Solid Edge part; units mm, degrees
sketch "Sketch1" plane through (0, 0, 0) normal (0, 0, 1) x (1, 0, 0)
  line L0 (45, 22.5) -> (-45, 22.5)
  line L1 (-45, -22.5) -> (45, -22.5)
  arc A0 (-45, -22.5) -> (-45, 22.5) centre (-45, 0) cw
  arc A1 (45, 22.5) -> (45, -22.5) centre (45, 0) cw
  circle A2 centre (-45, 0) radius 10
  circle A3 centre (45, 0) radius 10
extrude "Protrusion1" add sketch "Sketch1" against normal blind 15
sketch "Sketch2" plane through (0, 0, 0) normal (1, 0, 0) x (0, 1, 0)
  line L0 (-7.5, 55) -> (-22.5, 0)
  line L1 (-22.5, 0) -> (0, 0)
  line L2 (0, 0) -> (0, 55)
  line L3 (0, 55) -> (-7.5, 55)
extrude "ExtrudedProtrusion_2" add sketch "Sketch2" along normal mid plane 15
sketch "Sketch3" plane through (0, 0, 0) normal (0, -1, 0) x (1, 0, 0)
  line L0 (15, 55) -> (24.5, 0)
  line L1 (0, 0) -> (24.5, 0)
  line L2 (0, 0) -> (-24.5, 0)
  line L3 (-15, 55) -> (-24.5, 0)
  line L4 (0, 55) -> (-15, 55)
  line L5 (0, 55) -> (15, 55)
extrude "ExtrudedProtrusion_3" add sketch "Sketch3" against normal blind 22.5
sketch "Sketch4" plane through (0, 7.5, 55) normal (0, 0, 1) x (0, 1, 0)
  line L0 (-15, 15) -> (-15, -15)
  line L1 (-15, -15) -> (15, -15)
  line L2 (15, -15) -> (15, 15)
  line L3 (15, 15) -> (-15, 15)
extrude "ExtrudedProtrusion_4" add sketch "Sketch4" along normal blind 30
sketch "Sketch5" plane through (0, -7.5, 70) normal (0, -1, 0) x (1, 0, 0)
  line L0 (10, -10) -> (10, 10)
  line L1 (10, 10) -> (-10, 10)
  line L2 (-10, 10) -> (-10, -10)
  line L3 (-10, -10) -> (10, -10)
extrude "ExtrudedCutout_1" cut sketch "Sketch5" along normal mid plane 100
sketch "Sketch6" plane through (15, 7.5, 70) normal (1, 0, 0) x (0, 1, 0)
  line L0 (5, -12) -> (5, 12)
  line L1 (5, 12) -> (-5, 12)
  line L2 (-5, 12) -> (-5, -12)
  line L3 (-5, -12) -> (5, -12)
extrude "ExtrudedProtrusion_5" add sketch "Sketch6" along normal blind 25
sketch "Sketch7" plane through (-15, 7.5, 70) normal (-1, 0, 0) x (0, 0, 1)
  line L0 (-12, 5) -> (12, 5)
  line L1 (12, 5) -> (12, -5)
  line L2 (12, -5) -> (-12, -5)
  line L3 (-12, -5) -> (-12, 5)
extrude "ExtrudedProtrusion_6" add sketch "Sketch7" along normal blind 25
sketch "Sketch8" plane through (27.5, 2.5, 70) normal (0, -1, 0) x (1, 0, 0)
  circle A0 centre (12.5, 0) radius 5
extrude "ExtrudedCutout_3" cut sketch "Sketch8" along normal mid plane 50
sketch "Sketch9" plane through (27.5, 2.5, 70) normal (0, -1, 0) x (1, 0, 0)
  circle A0 centre (12.5, 0) radius 12
  circle A1 centre (12.5, 0) radius 5
extrude "ExtrudedProtrusion_7" add sketch "Sketch9" against normal blind 10
sketch "Sketch10" plane through (-27.5, 2.5, 70) normal (0, -1, 0) x (1, 0, 0)
  circle A0 centre (-12.5, 0) radius 12
  circle A1 centre (-12.5, 0) radius 5
extrude "ExtrudedProtrusion_8" add sketch "Sketch10" against normal blind 10
sketch "Sketch11" plane through (-27.5, 2.5, 70) normal (0, -1, 0) x (1, 0, 0)
  circle A0 centre (-12.5, 0) radius 5
extrude "ExtrudedCutout_5" cut sketch "Sketch11" along normal mid plane 50
fillet "Round_2" radius 3 4 edges at (15, 7.5, 82) (-15, 7.5, 82) (15, 7.5, 58) (-15, 7.5, 58)
Here's how the part is built. I have some questions about the finished solid (model axes, mm). A direction names the side the tool comes from. Coordinates: 2 decimals unless noted, no trailing zeros. Loops run counter-clockwise (first coordinate to the right, second up) from the corner with the lowest first, then second, coordinate; pieces in that order, holes last. Notation, with made-up numbers: (30, -2.75) -> (41, -2.75) arc R23 cw to (41, 29.25) -> close; hole circle Ø11 at (-5.5, -5). An arc over 180 degrees is marked (long way). Use one line per item in the form item = value. Start each with the question number.
(1) We'd pull the mould along X, two halves only. Please class faces 4 (the face through (-15, 1, 70)), 5 (the face through (-10, 8, 70)), 6 (the face through (33, 2.5, 70)): pulls with the +X half, pulls with the -X half, needs draft (parallel to the pull), parting line crosses it, or undercut.
(2) If we section it at B-B (y = -6): Please give me the cut outline in (x, z), then the cut area to 3 significant figures.
(3) If we section it at D-D (z = 6.5): Please give me the cut outline in (x, y), then the cut area to 3 significant figures.
(4) If we section it at A-A (x = -1.5): Please give me the cut outline in (y, z).
(5) Please list where these lines run through material, in increasing order: line 1 along X through (y, z) = (8, 70); line 2 along X through (y, z) = (2, 65); line 3 along Y through (x, z) = (-45, -4).
(6) On a 3-axis mill with a long thin cutter (end or side, diameter ignored), from which of +Z, -Z, +X, -X, +Y, -Y can I reach the whole of each face in a straight line? I mean faces 1 (the face through (11, -4, 55)), 2 (the face through (19.683, 11.092, 27.885)), 3 (the face through (29, 8, 82)). Say none if no direction works.
(7) Will these pins go through, and if not, where does the flat tip stop? pin 1 (24 mm diameter, centred on x = -40.5, z = 68.5, fed in from +Y); pin 2 (22 mm diameter, centred on y = 9, z = 68, fed in from -X); pin 3 (3 mm diameter, centred on y = 7.5, z = 38.5, fed in from +X).
(8) If we section it at C-C (x = -37): Please give me the cut outline in (y, z).
Verdict:
q1.face_4 = pulls with the -X half
q1.face_5 = undercut
q1.face_6 = needs draft
q2.outline = (-66.69, -15) -> (-53, -15) -> (-53, 0) -> (-66.69, 0) -> close; (-37, -15) -> (37, -15) -> (37, 0) -> (7.5, 0) -> (7.5, 55) -> (15, 55) -> (15, 85) -> (-15, 85) -> (-15, 55) -> (-7.5, 55) -> (-7.5, 0) -> (-37, 0) -> close; (53, -15) -> (66.69, -15) -> (66.69, 0) -> (53, 0) -> close; hole (-10, 60) -> (10, 60) -> (10, 80) -> (-10, 80) -> close
q2.area = 2,850 mm²
q3.outline = (-23.38, 0) -> (-7.5, 0) -> (-7.5, -20.73) -> (7.5, -20.73) -> (7.5, 0) -> (23.38, 0) -> (23.38, 22.5) -> (-23.38, 22.5) -> close
q3.area = 1,360 mm²
q4.outline = (-22.5, -15) -> (22.5, -15) -> (22.5, 60) -> (-7.5, 60) -> (-7.5, 55) -> (-22.5, 0) -> close; (-7.5, 80) -> (22.5, 80) -> (22.5, 85) -> (-7.5, 85) -> close
q5.line_1 = -52 to -45, -35 to -10, 10 to 35, 45 to 52
q5.line_2 = -15 to -10, 10 to 15
q5.line_3 = -22.5 to -10, 10 to 22.5
q6.face_1 = +X, -Y
q6.face_2 = +X, +Y, -Y
q6.face_3 = +Z, +X, +Y, -Y
q7.pin_1 = 12.5
q7.pin_2 = -52
q7.pin_3 = 18.11
q8.outline = (-22.5, -15) -> (-6, -15) -> (-6, 0) -> (-22.5, 0) -> close; (2.5, 58) -> (12.5, 58) -> (12.5, 66) -> (2.5, 66) -> close; (2.5, 74) -> (12.5, 74) -> (12.5, 82) -> (2.5, 82) -> close; (6, -15) -> (22.5, -15) -> (22.5, 0) -> (6, 0) -> close
